Study the drawing (mm; zero at the part's minimum x, y, z) and answer. A direction names the side the tool comes from. Coordinates: 2 decimals unless noted, no trailing zeros. Loops run counter-clockwise (first coordinate to the right, second up) from the corner with the lowest first, then second, coordinate; pieces in that order, holes last. Notation, with made-up numbers: (60, 54.5) - (84, 54.5) arc R26 ccw to (84, 87.5) - close; hole circle Ø2 at (21.5, 83). An arc over 180 degrees is marked (long way). Write each question's results on one line, items separated by ' | '. Start each with the question number.
(1) Find section C-C on x = 35. Determine the outline of the cut face in (y, z).
(2) Determine the mould class of the marked faces 1, 2 and 3 for opening direction X: released by +X, released by -X, zero draft, split by the parting line, or undercut.
(3) Find section A-A on y = 18.5. Determine the outline of the cut face in (x, z), then the cut area to 3 significant figures.
(4) Given pin 1 Ø11.5 at (x, y) = (32, 17) entering from -Z, flat-ended and moving along its own axis, determine where the tip first touches the part or whether it passes through.
(5) Find section B-B on z = 5. Determine the outline of the cut face in (x, y), then the cut area to 3 significant figures.
(6) Find section D-D on y = 13.25. Determine the outline of the cut face in (x, z).
(7) For the marked faces 4, 5, 6, 7 and 8, determine the directions among +Z, -Z, +X, -X, +Y, -Y from which every point of the face is accessible in a straight line to the end or side of a thin tool.
(8) Consider line 1 (Z direction, x = 29, y = 17.5); line 2 (X direction, y = 16.75, z = 22); line 3 (Z direction, x = 5.5, y = 9.25). Determine where each line is inside the solid, lowest interval first. Write a range as from..to.
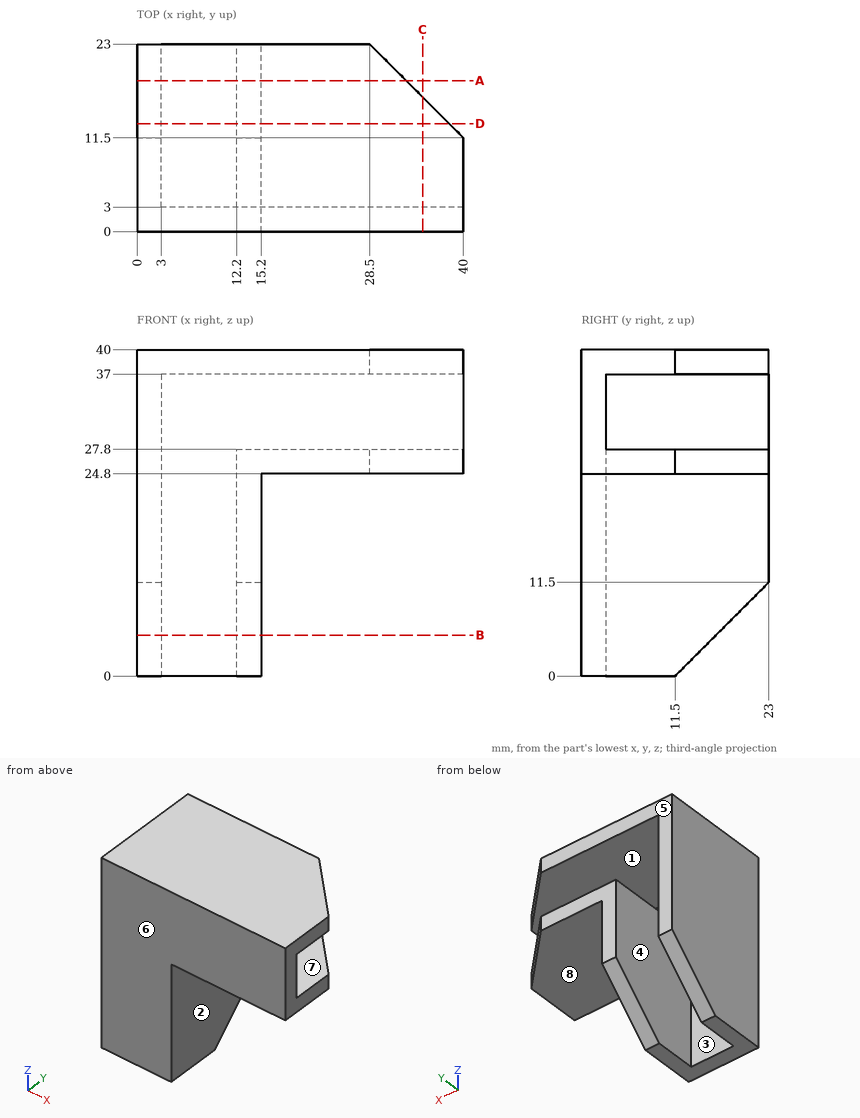
Values:
1) outline: (0, 24.8) - (16.5, 24.8) - (16.5, 27.8) - (3, 27.8) - (3, 37) - (16.5, 37) - (16.5, 40) - (0, 40) - close
2) face 1: zero draft | face 2: released by +X | face 3: undercut
3) outline: (0, 7) - (3, 7) - (3, 37) - (33, 37) - (33, 40) - (0, 40) - close; (12.2, 7) - (15.2, 7) - (15.2, 24.8) - (33, 24.8) - (33, 27.8) - (12.2, 27.8) - close | area: 305 mm²
4) pin 1: stops at z = 24.8
5) outline: (0, 0) - (15.2, 0) - (15.2, 16.5) - (12.2, 16.5) - (12.2, 3) - (3, 3) - (3, 16.5) - (0, 16.5) - close | area: 127 mm²
6) outline: (0, 1.75) - (3, 1.75) - (3, 37) - (38.25, 37) - (38.25, 40) - (0, 40) - close; (12.2, 1.75) - (15.2, 1.75) - (15.2, 24.8) - (38.25, 24.8) - (38.25, 27.8) - (12.2, 27.8) - close
7) face 4: -Z, +Y | face 5: +Z, -Z, +X, -X, +Y | face 6: +Z, -Z, +X, -X, -Y | face 7: +X, +Y | face 8: -Z, +X, +Y, -Y
8) line 1: z = 24.8..27.8, 37..40 | line 2: x = 0..3, 12.2..15.2 | line 3: z = 37..40
